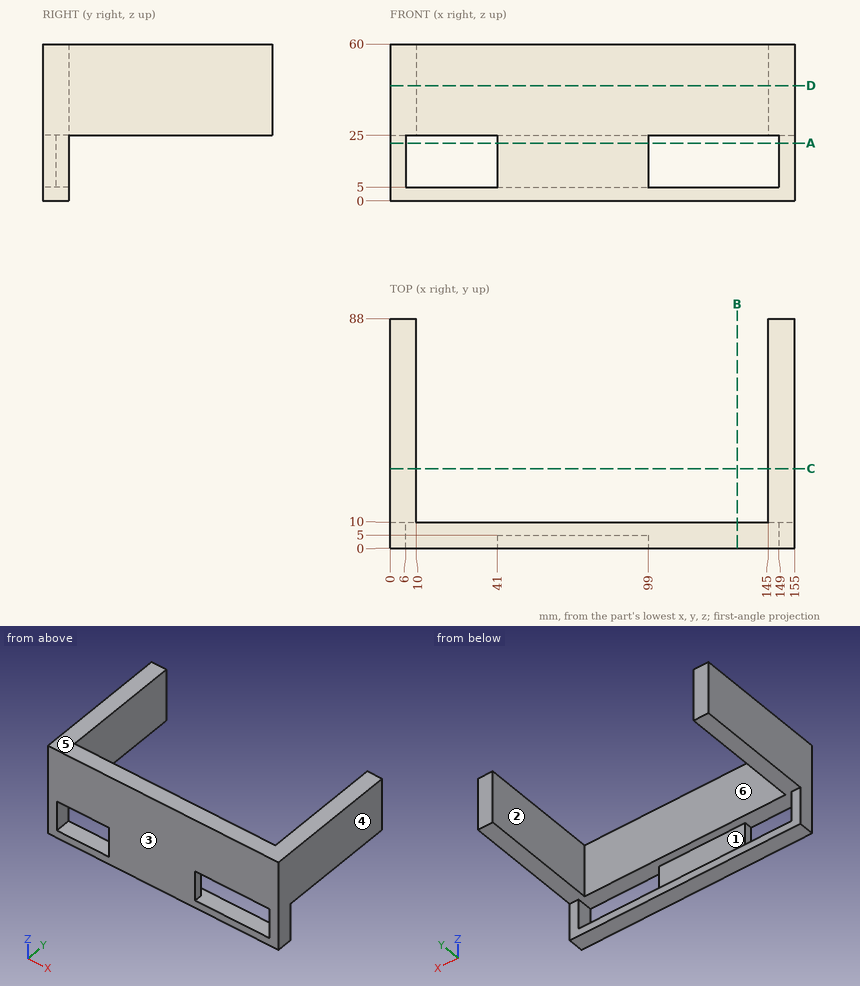
Can you work these out from the drawing? Everything is in mm from the part's minimum corner. A direction names the side the tool comes from. Coordinates: 2 decimals unless noted, no trailing zeros. Loops run counter-clockwise (first coordinate to the right, second up) from the corner with the lowest first, then second, coordinate; pieces in that order, holes last.
1) Will these pins go through, and if not, where does the flat tip stop? pin 1 Ø6 at (x, z) = (63, 17.5) entering from +Y; pin 2 Ø6 at (x, z) = (72.5, 23) entering from +Y.
Reported:
pin 1: stops at y = 5
pin 2: stops at y = 10
2) Imagine slicing it at A-A (z = 22). List the corners of the cut face in (x, y) for me.
Reported:
outline: (0, 0) - (6, 0) - (6, 10) - (0, 10) - close; (41, 0) - (99, 0) - (99, 5) - (41, 5) - close; (149, 0) - (155, 0) - (155, 10) - (149, 10) - close
3) Imagine slicing it at B-B (x = 133). List the corners of the cut face in (y, z) for me, and give its area (3 significant figures).
Reported:
outline: (0, 0) - (10, 0) - (10, 5) - (0, 5) - close; (0, 25) - (10, 25) - (10, 60) - (0, 60) - close
area: 400 mm2
4) Which directions (+Z, -Z, +X, -X, +Y, -Y) give clear straight access to the entire face, cutting with the end or side of a thin tool? Please do the marked faces 1, 2 and 3.
Reported:
face 1: +Y
face 2: +Z, -Z, +Y
face 3: +Z, -Z, +X, -X, -Y
5) Thinking about a two-plate mould opening in X: for the marked faces 4, 5 and 6, which applies, released by +X, released by -X, zero draft, split by the parting line, or undercut?
Reported:
face 4: released by +X
face 5: zero draft
face 6: undercut
6) Imagine slicing it at D-D (z = 44). List the corners of the cut face in (x, y) for me.
Reported:
outline: (0, 0) - (155, 0) - (155, 88) - (145, 88) - (145, 10) - (10, 10) - (10, 88) - (0, 88) - close
7) Please list where these lines run through material, in increasing order: line 1 along X through (y, z) = (30, 48); line 2 along Y through (x, z) = (52, 46); line 3 along Z through (x, y) = (148.5, 64.5).
Reported:
line 1: x = 0 to 10, 145 to 155
line 2: y = 0 to 10
line 3: z = 25 to 60
8) Imagine slicing it at C-C (y = 30.5). List the corners of the cut face in (x, z) for me.
Reported:
outline: (0, 25) - (10, 25) - (10, 60) - (0, 60) - close; (145, 25) - (155, 25) - (155, 60) - (145, 60) - close
